For this review, use the dimensioned drawing (mm, ordinates from the lowest corner) and the shaded views. Give positions to 0.01 mm unless a question says otherwise; leave off trailing zeros. Write each loop counter-clockwise with the first axis right and the second up, starting at its lowest first coordinate (ties: lowest second). Pieces come first, ordered by that corner, then holes.
1) Wall thickness on line 1 along X through (y, z) = (1.75, 3); line 2 along X through (y, z) = (2.7, 5.55); line 3 along X through (y, z) = (2.7, 2.6): over which ranges is each line inside the solid? List them lowest first.
2) For P1, Ø1.8, axis at x = 3, z = 3, coming from the -Y side; P2, Ø1.5, axis at x = 19, y = 1, coming from the +Z side; P3, Ø1.5, axis at x = 20, y = 1, coming from the -Z side; P4, Ø3, axis at x = 33.5, z = 2.5, coming from the -Y side, all flat-tipped, find the tip position at first contact; note any pin that passes through.
3) We need section C-C on y = 1.95. Give the boundary of the cut face in (x, z), and give its area (3 significant figures).
4) Draft analysis for pull direction X (two halves, no side actions). For the marked faces 1 and 2, state which applies: pulls with the +X half, pulls with the -X half, needs draft (parallel to the pull), parting line crosses it, or undercut.
5) We need section D-D on x = 16. Give the boundary of the cut face in (y, z), and give its area (3 significant figures).
6) We need section A-A on x = 28. Give the boundary of the cut face in (y, z).
7) We need section B-B on z = 5.4. Give the boundary of the cut face in (x, y), and give its area (3 significant figures).
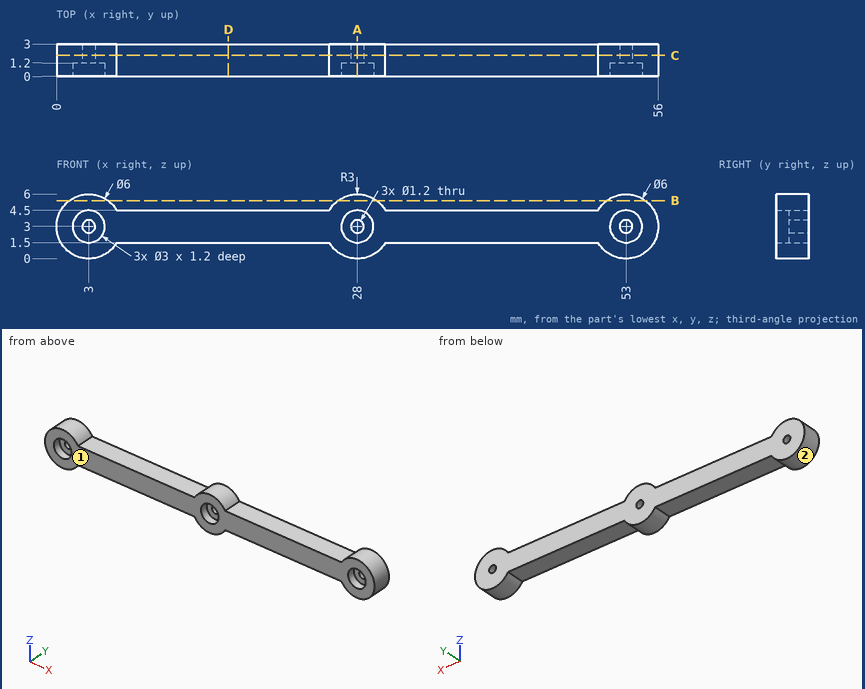
Results list:
1. line 1: x = 0 to 2.4, 3.6 to 27.4, 28.6 to 52.4, 53.6 to 56
1. line 2: x = 1.42 to 4.58, 26.42 to 29.58, 51.42 to 54.58
1. line 3: x = 0.03 to 2.55, 3.45 to 27.55, 28.45 to 52.55, 53.45 to 55.97
2. P1: stops at y = 1.2
2. P2: stops at z = 4.5
2. P3: stops at z = 1.5
2. P4: stops at y = 0
3. outline: (5.6, 1.5) - (25.4, 1.5) arc R3 ccw to (30.6, 1.5) - (50.4, 1.5) arc R3 ccw (long way) to (50.4, 4.5) - (30.6, 4.5) arc R3 ccw to (25.4, 4.5) - (5.6, 4.5) arc R3 ccw (long way) to start; hole circle Ø1.2 at (3, 3); hole circle Ø1.2 at (28, 3); hole circle Ø1.2 at (53, 3)
3. area: 197 mm2
4. face 1: needs draft
4. face 2: undercut
5. outline: (0, 1.5) - (3, 1.5) - (3, 4.5) - (0, 4.5) - close
5. area: 9.00 mm2
6. outline: (0, 0) - (3, 0) - (3, 2.4) - (1.2, 2.4) - (1.2, 1.5) - (0, 1.5) - close; (0, 4.5) - (1.2, 4.5) - (1.2, 3.6) - (3, 3.6) - (3, 6) - (0, 6) - close
7. outline: (1.2, 0) - (4.8, 0) - (4.8, 3) - (1.2, 3) - close; (26.2, 0) - (29.8, 0) - (29.8, 3) - (26.2, 3) - close; (51.2, 0) - (54.8, 0) - (54.8, 3) - (51.2, 3) - close
7. area: 32.4 mm2
